Can you work these out from the model? Positions are in its coordinate system, mm. A direction names the side the tool comes from. Coordinates: 2 decimals unless noted, no trailing zeros. Loops run counter-clockwise (first coordinate to the right, second up) from the corner with the lowest first, then second, coordinate; pieces in that order, holes last. Notation, with made-up numbers: M 86.5,69.5 L 102.5,69.5 A12 cw 102.5,77.5 Z; hole C 68,-28 d6. An arc over 180 degrees is marked long. Answer as a JSON object with one key per item and string values. Group by question number.
Item 1: If I drill on line 1 (Y direction, x = 2.45, z = -30.1); line 2 (Y direction, x = 9.75, z = -9); line 3 (Y direction, x = 3.75, z = -30), over which ranges is the centre line in solid material (lowest first)?
Item 2: Suppose I cut it at C-C (y = 29.5). Write out the boundary of the cut face in (x, z).
Item 3: Suppose I cut it at D-D (y = 42.5). Write out the boundary of the cut face in (x, z).
Item 4: Suppose I cut it at B-B (z = -22.1). Write out the boundary of the cut face in (x, y).
Item 5: We'd pull the mould along Y, two halves only. Please class faces 4 (the flat face through (10, 4, -76.2)), 5 (the cylindrical face through (1.93, 38.2, -29.43)), 6 (the cylindrical face through (1.9, 38.4, -38.2)), 7 (the flat face through (10, 0, -38)): +Y half, -Y half, draft (parallel to the pull), parting line (faces both ways), or undercut.
Item 6: I'm going to push flat-ended pins straight in: pin 1 Ø3 at (y, z) = (11.54, -30.1) entering from +X; pin 2 Ø1.5 at (x, y) = (3.5, 18.5) entering from +Z; pin 3 Ø3 at (x, z) = (10.5, -7) entering from +Y. Where does each tip first touch, or does it pass through?
Item 7: Which directions (+Z, -Z, +X, -X, +Y, -Y) give clear straight access to the entire face, cutting with the end or side of a thin tool? Please do faces 1 (the cylindrical face through (11.107, 10.471, -65.023)), 2 (the flat face through (3.81, 13, -42)), 3 (the cylindrical face through (1.9, 32, -26.9)).
Autodesk Inventor part; units mm, degrees
ref_plane "YZ Plane" through (0, 0, 0) normal (1, 0, 0) x (0, 1, 0)
ref_plane "XZ Plane" through (0, 0, 0) normal (0, 1, 0) x (-1, 0, 0)
ref_plane "XY Plane" through (0, 0, 0) normal (0, 0, 1) x (1, 0, 0)
sketch "Sketch1" plane through (0, 0, 0) normal (0, 1, 0) x (-1, 0, 0)
  line L0 (0, 0) -> (-19.05, 0)
  line L1 (-19.05, 0) -> (-19.05, -76.2)
  line L2 (-19.05, -76.2) -> (0, -76.2)
  line L3 (0, -76.2) -> (0, 0)
  dimension "d0" = 19.05
  dimension "d1" = 76.2
extrude "Extrusion1" add sketch "Sketch1" along normal blind 7.62
sketch "Sketch2" plane through (0, 7.62, 0) normal (0, 1, 0) x (1, 0, 0)
  line L0 (0, 0) -> (0, 12.7)
  line L1 (0, 12.7) -> (19.05, 12.7)
  line L2 (19.05, 12.7) -> (19.05, 63.5)
  line L3 (19.05, 63.5) -> (0, 63.5)
  line L4 (0, 63.5) -> (0, 12.7)
  dimension "d4" = 12.7
  dimension "d5" = 19.05
  dimension "d6" = 50.8
extrude "Extrusion2" add sketch "Sketch2" along normal blind 43.18
sketch "Sketch3" plane through (19.05, 0, 0) normal (1, 0, 0) x (0, 0, -1)
  line L0 (12.7, 50.8) -> (63.5, 50.8)
  line L1 (38.1, 50.8) -> (38.1, 25.4)
  circle A0 centre (38.1, 25.4) radius 18.542
  point P0 (0, 0)
  dimension "d9" = 25.4
  dimension "d10" = 37.084
extrude "Extrusion3" cut sketch "Sketch3" against normal blind 15.24
fillet "Fillet1" radius 25.4 2 edges at (9.525, 50.8, -63.5) (9.525, 50.8, -12.7)
sketch "Sketch6" plane through (0, 7.62, 0) normal (0, 1, 0) x (1, 0, 0)
  line L0 (0, 0) -> (19.05, 0)
  line L1 (9.525, 0) -> (9.525, 6.35)
  line L2 (19.05, 76.2) -> (0, 76.2)
  line L3 (9.525, 76.2) -> (9.525, 69.85)
  dimension "d20" = 6.35
  dimension "d21" = 6.35
fillet "Fillet2" radius 25.4 2 edges at (9.525, 7.62, -63.5) (9.525, 7.62, -12.7)
hole "Hole1" at (9.525, 7.62, -6.35) at (9.525, 7.62, -69.85) direction (0, -1, 0) diameter 5.08 end through all counterbore diameter 10.16 counterbore depth 3.81
sketch "Sketch7" plane through (9.525, 7.62, -6.35) normal (0, -1, 0) x (1, 0, 0)
  circle A0 centre (0, 0) radius 5.08
  circle A1 centre (0, -63.5) radius 2.54
  line L0 (-2.54, -63.5) -> (0, -63.5)
  circle A2 centre (0, -63.5) radius 5.08
  point P0 (-9.525, 6.35)
  dimension "d30" = 10.16
  dimension "d31" = 10.16
extrude "Extrusion5" cut sketch "Sketch7" against normal blind 15.24 contours A0 | A1 | A2
sketch "Sketch10" plane through (3.81, 25.4, -38.1) normal (1, 0, 0) x (0, 0, -1)
  circle A0 centre (0, 0) radius 18.542
  circle A1 centre (-8, -13.8564) radius 1.25
  circle A2 centre (0, 7) radius 6
  circle A3 centre (16, 0) radius 1.25
  circle A4 centre (8, -13.8564) radius 1.25
  circle A5 centre (-16, 0) radius 1.25
  circle A6 centre (8, -13.8564) radius 1.25
  circle A7 centre (-8, -13.8564) radius 1.25
  circle A8 centre (-8, -13.8564) radius 1.25
  circle A9 centre (-16, 0) radius 1.25
  circle A10 centre (16, 0) radius 1.25
  point P0 (-38.1, -25.4)
extrude "Extrusion8" cut sketch "Sketch10" against normal blind 25.4 contours A1 | A2 | A3 | A4 | A5
pattern_circular "Circular Pattern4" count 6 over 360 about axis through (19.05, 25.4, -38.1) along (-1, 0, 0) of "Extrusion8"
sketch "Sketch14" plane through (3.81, 0, 0) normal (1, 0, 0) x (0, 0, -1)
  arc A0 (36.735, 25.4) -> (37.4175, 26.5821) centre (31.9408, 28.956) ccw
  arc A1 (37.4175, 24.2179) -> (36.735, 25.4) centre (31.9408, 21.844) ccw
  arc A2 (38.7825, 24.2179) -> (37.4175, 24.2179) centre (38.1, 18.288) ccw
  arc A3 (39.465, 25.4) -> (38.7825, 24.2179) centre (44.2592, 21.844) ccw
  arc A4 (38.7825, 26.5821) -> (39.465, 25.4) centre (44.2592, 28.956) ccw
  arc A5 (37.4175, 26.5821) -> (38.7825, 26.5821) centre (38.1, 32.512) ccw
  line L0 (38.7825, 24.2179) -> (37.4175, 24.2179)
  line L1 (37.4175, 24.2179) -> (36.735, 25.4)
  line L2 (36.735, 25.4) -> (37.4175, 26.5821)
  line L3 (37.4175, 26.5821) -> (38.7825, 26.5821)
  line L4 (38.7825, 26.5821) -> (39.465, 25.4)
  line L5 (39.465, 25.4) -> (38.7825, 24.2179)
  point P0 (0, 0)
  point P1 (38.1, 25.4)
extrude "Extrusion10" cut sketch "Sketch14" against normal blind 25.4 contours A0 A5 A4 A3 A2 A1
properties part number "Motor Mount V2"
From the geometry:
{
 "1": {"line 1": "0 to 10.29, 12.79 to 16.22, 34.58 to 38.01, 40.51 to 49.51", "line 2": "0 to 3.81", "line 3": "0 to 10.3, 12.79 to 16.26, 34.54 to 38.01, 40.5 to 49.47"},
 "2": {"outline": "M 0,-63.17 L 19.05,-63.17 L 19.05,-56.18 L 3.81,-56.18 L 3.81,-50.13 L 0,-50.13 Z; M 0,-26.07 L 3.81,-26.07 L 3.81,-20.02 L 19.05,-20.02 L 19.05,-13.03 L 0,-13.03 Z"},
 "3": {"outline": "M 0,-56.88 L 19.05,-56.88 L 19.05,-45.27 L 3.81,-45.27 L 3.81,-30.93 L 19.05,-30.93 L 19.05,-19.32 L 0,-19.32 Z"},
 "4": {"outline": "M 0,0 L 19.05,0 L 19.05,16.03 L 3.81,16.03 L 3.81,24.15 L 0,24.15 Z; M 0,26.65 L 3.81,26.65 L 3.81,34.77 L 19.05,34.77 L 19.05,45.13 L 0,45.13 Z"},
 "5": {"face 4": "draft", "face 5": "undercut", "face 6": "undercut", "face 7": "-Y half"},
 "6": {"pin 1": "x = 3.81", "pin 2": "z = -9.89", "pin 3": "y = 3.81"},
 "7": {"face 1": "+Y", "face 2": "+X", "face 3": "+X, -X"}
}
